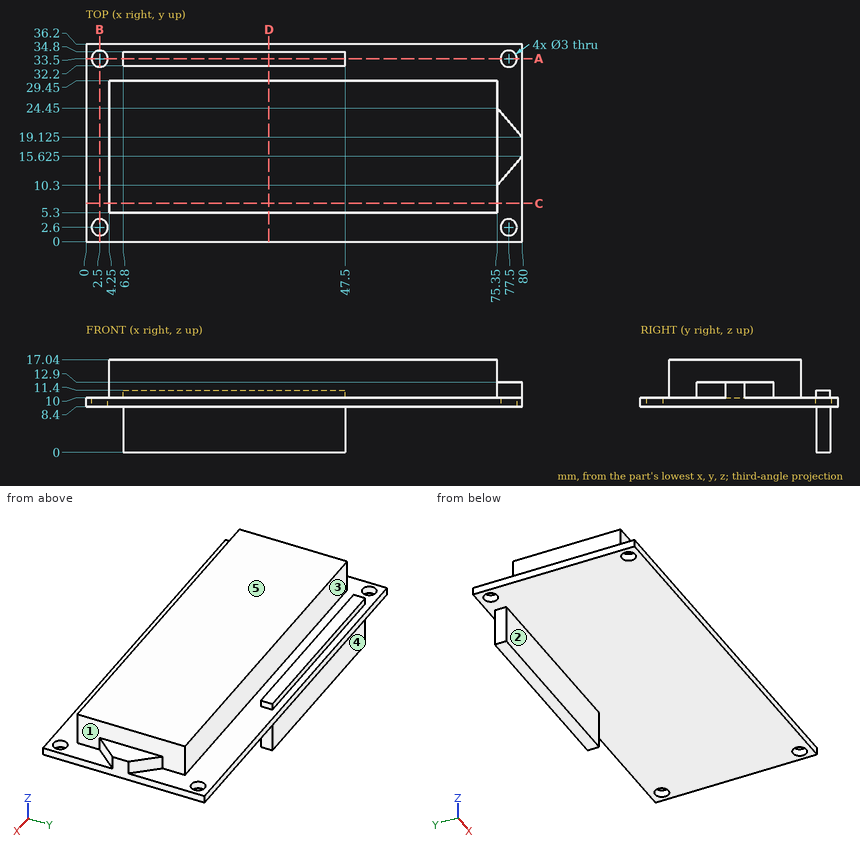
The drawing under review shows one solid part. Ordinate dimensions are in mm from its lowest x, y, z. A direction names the side the tool comes from. Give positions to 0.01 mm unless a question says otherwise; leave off trailing zeros. Order: outer loops, then holes, each group sorted by start corner. A loop starts at its lowest first (then second) coordinate and runs counter-clockwise, first axis right, second up. Notation, with made-up numbers: (38.25, -6) - (52.25, -6) arc R32 ccw to (52.25, 30) - close; hole circle Ø3 at (13, 25). An arc over 180 degrees is marked (long way). Answer as a JSON object with one key per item and string values. Group by question number.
Item 1: Clearance check with flat-ended pins moving along their axes: pin 1 Ø0.8 at (y, z) = (34, 4) entering from +X; pin 2 Ø3.5 at (x, y) = (77.5, 19.5) entering from +Z; pin 3 Ø5 at (x, y) = (77.5, 33.5) entering from +Z. State where each tip first meets the part, or that it passes through.
Item 2: Take a section at D-D on x = 33.5. Give the boundary of the cut face in (y, z), and give its area (3 significant figures).
Item 3: Take a section at B-B on x = 2.5. Give the boundary of the cut face in (y, z), and give its area (3 significant figures).
Item 4: Take a section at C-C on y = 7. Give the boundary of the cut face in (x, z), and give its area (3 significant figures).
Item 5: Machinability: for the marked faces 1, 2, 3, 4 and 5, which of the approach directions +Z, -Z, +X, -X, +Y, -Y give a long, thin tool a straight path to every point of the face, cutting with its end or side? Answer none if there is none.
Item 6: Wall thickness on line 1 along Y through (x, z) = (2.5, 9); line 2 along Y through (x, z) = (20, 10.5); line 3 along Z through (x, y) = (63, 19.5): over which ranges is each line inside the solid? List them lowest first.
Item 7: Take a section at A-A on y = 33.5. Give the boundary of the cut face in (x, z).
Reported:
{
 "1": {"pin 1": "x = 47.5", "pin 2": "z = 12.9", "pin 3": "z = 10"},
 "2": {"outline": "(0, 8.4) - (32.2, 8.4) - (32.2, 0) - (34.8, 0) - (34.8, 8.4) - (36.2, 8.4) - (36.2, 10) - (34.8, 10) - (34.8, 11.4) - (32.2, 11.4) - (32.2, 10) - (29.45, 10) - (29.45, 17.04) - (5.3, 17.04) - (5.3, 10) - (0, 10) - close", "area": "253 mm^2"},
 "3": {"outline": "(0, 8.4) - (1.1, 8.4) - (1.1, 10) - (0, 10) - close; (4.1, 8.4) - (32, 8.4) - (32, 10) - (4.1, 10) - close; (35, 8.4) - (36.2, 8.4) - (36.2, 10) - (35, 10) - close", "area": "48.3 mm^2"},
 "4": {"outline": "(0, 8.4) - (80, 8.4) - (80, 10) - (75.35, 10) - (75.35, 17.04) - (4.25, 17.04) - (4.25, 10) - (0, 10) - close", "area": "629 mm^2"},
 "5": {"face 1": "+Z, +X", "face 2": "-Z, +X, -X, -Y", "face 3": "+Z, +X, -X", "face 4": "-Z, +X, -X, +Y", "face 5": "+Z, +X, -X, +Y, -Y"},
 "6": {"line 1": "0 to 1.1, 4.1 to 32, 35 to 36.2", "line 2": "5.3 to 29.45, 32.2 to 34.8", "line 3": "8.4 to 17.04"},
 "7": {"outline": "(0, 8.4) - (1, 8.4) - (1, 10) - (0, 10) - close; (4, 8.4) - (6.8, 8.4) - (6.8, 0) - (47.5, 0) - (47.5, 8.4) - (76, 8.4) - (76, 10) - (47.5, 10) - (47.5, 11.4) - (6.8, 11.4) - (6.8, 10) - (4, 10) - close; (79, 8.4) - (80, 8.4) - (80, 10) - (79, 10) - close"}
}
